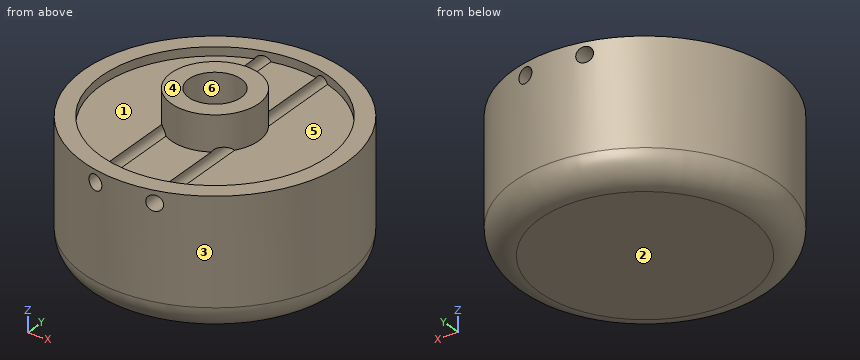
```python
from build123d import *

# Parameters (mm, degrees)
F0_R           = 15
F1_DEPTH       = 15
F2_R           = 13
F3_DEPTH       = 1
F4_R           = 5
F5_DEPTH       = 4
F6_R           = 3
F7_DEPTH       = 13
F8_R           = 3
F9_R           = 0.875
F10_DEPTH      = 15.001
F10_DEPTH_BACK = 15.001


with BuildPart() as f1:
    # F0 (on Top) → F1 (new body)
    with BuildSketch(Plane.XY):
        Circle(F0_R)
    extrude(amount=F1_DEPTH)

    # F2 (on face) → F3 (cut)
    with BuildSketch(Plane.XY.offset(15)):
        Circle(F2_R)
    extrude(amount=-F3_DEPTH, mode=Mode.SUBTRACT)

    # F4 (on face) → F5 (join)
    with BuildSketch(Plane.XY.offset(14)):
        Circle(F4_R)
    extrude(amount=F5_DEPTH)

    # F6 (on face) → F7 (cut)
    with BuildSketch(Plane.XY.offset(18)):
        Circle(F6_R)
    extrude(amount=-F7_DEPTH, mode=Mode.SUBTRACT)

    # F8
    f8_edges = [f1.edges().sort_by_distance(p)[0] for p in [
        (-15, 0, 0),
    ]]
    fillet(f8_edges, radius=F8_R)

    # F9 (on Front) → F10 (cut, two sides)
    with BuildSketch(Plane.XZ) as f10_sk:
        with Locations((-3.375, 13.625)):
            Circle(F9_R)
        with Locations((3.375, 13.625)):
            Circle(F9_R)
    extrude(amount=-F10_DEPTH, mode=Mode.SUBTRACT)
    extrude(f10_sk.sketch, amount=F10_DEPTH_BACK, mode=Mode.SUBTRACT)


solid = f1.part
```
Can you work these out from the model? Positions are in its coordinate system, mm. Face numbers are marked on the shaded views. A direction names the side the tool comes from. Coordinates: 2 decimals unless noted, no trailing zeros. Write each loop counter-clockwise with the first axis right and the second up, starting at its lowest first coordinate (ties: lowest second). Pieces come first, ordered by that corner, then holes. Notation, with made-up numbers: (43.5, -24) - (59.5, -24) arc R29 cw to (59.5, -4) - close; hole circle Ø6 at (69.5, 31.25). An arc over 180 degrees is marked (long way). Return JSON: item names as keys, results as strings.
Q1. On a 3-axis mill with a long thin cutter (end or side, diameter ignored), from which of +Z, -Z, +X, -X, +Y, -Y can I reach the whole of each face in a straight line? I mean the marked faces 1 and 2. Say none if no direction works.
Computed values:
{"face 1": "+Z", "face 2": "-Z, +X, -X, +Y, -Y"}
Q2. I'm going to push flat-ended pins straight in: pin 1 Ø2.5 at (x, y) = (-1, 9.5) entering from +Z; pin 2 Ø4 at (x, z) = (-4.5, 3.5) entering from -Y; pin 3 Ø1.8 at (x, y) = (0.5, 0.5) entering from +Z. Where does each tip first touch, or does it pass through?
Computed values:
{"pin 1": "stops at z = 14", "pin 2": "stops at y = -14.79", "pin 3": "stops at z = 5"}
Q3. If we section it at B-B (z = 10): Please give me the cut outline in (x, y), then the cut area to 3 significant figures.
Computed values:
{"outline": "circle Ø30 at (0, 0); hole circle Ø6 at (0, 0)", "area": "679 mm2"}
Q4. Thinking about a two-plate mould opening in Y: for the marked faces 3, 4, 5 and 6, which applies, +Y half, -Y half, draft (parallel to the pull), parting line (faces both ways), or undercut?
Computed values:
{"face 3": "parting line", "face 4": "draft", "face 5": "undercut", "face 6": "undercut"}
Q5. If we section it at A-A (x = 0): Please give me the cut outline in (y, z), then the cut area to 3 significant figures.
Computed values:
{"outline": "(-15, 3) arc R3 ccw to (-12, 0) - (12, 0) arc R3 ccw to (15, 3) - (15, 15) - (13, 15) - (13, 14) - (5, 14) - (5, 18) - (3, 18) - (3, 5) - (-3, 5) - (-3, 18) - (-5, 18) - (-5, 14) - (-13, 14) - (-13, 15) - (-15, 15) - close", "area": "382 mm2"}
Q6. If we section it at C-C (z = 2.5): Please give me the cut outline in (x, y), then the cut area to 3 significant figures.
Computed values:
{"outline": "circle Ø29.92 at (0, 0)", "area": "703 mm2"}
Q7. Please list where these lines run through material, in increasing order: L1, parallel to X at y = 0, z = 15.75; L2, parallel to X at y = -7, z = 13; L3, parallel to X at y = -2, z = 13.25. Write a range as from..to.
Computed values:
{"L1": "x = -5..-3, 3..5", "L2": "x = -13.27..-3.99, -2.76..2.76, 3.99..13.27", "L3": "x = -14.87..-4.17, -2.58..-2.24, 2.24..2.58, 4.17..14.87"}
